Autodesk Inventor part; units mm, degrees
ref_plane "YZ Plane" through (0, 0, 0) normal (1, 0, 0) x (0, 1, 0)
ref_plane "XZ Plane" through (0, 0, 0) normal (0, 1, 0) x (-1, 0, 0)
ref_plane "XY Plane" through (0, 0, 0) normal (0, 0, 1) x (1, 0, 0)
sketch "Sketch1" plane through (0, 0, 0) normal (0, 0, 1) x (1, 0, 0)
  line L0 (0, 54.6) -> (0, -54.6)
  line L1 (-7.4, 0) -> (44.4, 0)
  line L2 (0, -39) -> (37, -39)
  line L3 (37, -39) -> (37, 39)
  line L4 (37, 39) -> (0, 39)
  line L5 (0, 39) -> (0, -39)
  dimension "d0" = 78
  dimension "d1" = 37
extrude "Extrusion1" add sketch "Sketch1" along normal blind 10
sketch "Sketch2" plane through (0, -39, 0) normal (-1, 0, 0) x (0, 0, 1)
  line L0 (10, 0) -> (10, 78)
  line L1 (0, 0) -> (10, 0)
  arc A0 (64.9146, 20.2333) -> (64.9146, 57.7667) centre (58, 39) ccw
  line L2 (10, 78) -> (64.9146, 57.7667)
  line L3 (10, 0) -> (64.9146, 20.2333)
  line L4 (10, 39) -> (96.3921, 39) construction
  dimension "d4" = 20
  dimension "d5" = 48
extrude "Extrusion2" add sketch "Sketch2" against normal blind 10
sketch "Sketch4" plane through (0, 0, 0) normal (0, 1, 0) x (-1, 0, 0)
  line L0 (-37, 10) -> (-10, 10)
  line L1 (-10, 10) -> (0, 10)
  line L2 (0, 0) -> (0, 10)
  line L3 (0, 0) -> (-37, 0)
  line L4 (-37, 0) -> (-37, 10)
  line L5 (-10, 10) -> (-10, 64.9146)
  line L6 (-10, 42) -> (-30, 10)
  line L7 (-10, 42) -> (-10, 10)
  line L8 (-10, 10) -> (-30, 10)
  dimension "d12" = 32
  dimension "d13" = 20
extrude "Extrusion3" add sketch "Sketch4" along normal mid plane 15 contours L6 L5 L0
properties part number "Bracket"
The listing builds one solid part. Answer for the finished solid, in the listing's coordinates (mm). A direction names the side the tool comes from. Coordinates: 2 decimals unless noted, no trailing zeros. Write each loop counter-clockwise with the first axis right and the second up, starting at its lowest first coordinate (ties: lowest second). Pieces come first, ordered by that corner, then holes.
Q1. Section D-D, the plane x = 31 is taken. Write down the section's boundary in (y, z), then the cut area to 3 significant figures.
Returned:
outline: (-39, 0) - (39, 0) - (39, 10) - (-39, 10) - close
area: 780 mm2
Q2. Given P1, Ø12, axis at x = 8, z = 35, coming from the +Y side; P2, Ø8, axis at x = 15, y = -22, coming from the +Z side; P3, Ø10, axis at x = 25, z = 27, coming from the +Y side, each flat-ended and moving along its own axis, determine where each tip first touches the part or whether it passes through.
Returned:
P1: stops at y = 32
P2: stops at z = 10
P3: stops at y = 7.5
Q3. Which of the six approach directions +Z, -Z, +X, -X, +Y, -Y give full straight-line access (tool end or side, diameter ignored) to faces 1 (the flat face through (16, 7.5, 19)), 2 (the flat face through (16, -7.5, 19)), 3 (the flat face through (10, 1, 44)), 4 (the cylindrical face through (5, 0, 78)), 5 (the flat face through (18, -39, 5))?
Returned:
face 1: +Z, +X, +Y
face 2: +Z, +X, -Y
face 3: +Z, +X
face 4: +Z, +X, -X
face 5: +Z, -Z, +X, -X, -Y
Q4. Find the intervals of material crossed by line 1 along X through (y, z) = (9.5, 66); line 2 along Y through (x, z) = (20.5, 12), in increasing order.
Returned:
line 1: x = 0 to 10
line 2: y = -7.5 to 7.5
Q5. Section B-B, the plane z = 21.5 is taken. Write down the section's boundary in (x, y).
Returned:
outline: (0, -34.76) - (10, -34.76) - (10, -7.5) - (22.81, -7.5) - (22.81, 7.5) - (10, 7.5) - (10, 34.76) - (0, 34.76) - close
Q6. Section A-A, the plane x = 12 is taken. Write down the section's boundary in (y, z).
Returned:
outline: (-39, 0) - (39, 0) - (39, 10) - (7.5, 10) - (7.5, 38.8) - (-7.5, 38.8) - (-7.5, 10) - (-39, 10) - close
Q7. Section C-C, the plane y = 33 is taken. Write down the section's boundary in (x, z).
Returned:
outline: (0, 0) - (37, 0) - (37, 10) - (10, 10) - (10, 26.28) - (0, 26.28) - close
